Autodesk Inventor part; units mm, degrees
ref_plane "YZ Plane" through (0, 0, 0) normal (1, 0, 0) x (0, 1, 0)
ref_plane "XZ Plane" through (0, 0, 0) normal (0, 1, 0) x (-1, 0, 0)
ref_plane "XY Plane" through (0, 0, 0) normal (0, 0, 1) x (1, 0, 0)
sketch "Sketch1" plane through (0, 0, 0) normal (0, 1, 0) x (-1, 0, 0)
  circle A0 centre (0, 0) radius 7.25
  circle A1 centre (0, 0) radius 5.5
  dimension "d0" = 14.5
  dimension "d7" = 11
sketch "Sketch2" plane through (0, 0, 0) normal (0, 0, 1) x (1, 0, 0)
  line L0 (0, 0) -> (0, 23) construction
  line L1 (0, 23) -> (3, 23) construction
  line L2 (3, 23) -> (3, 46) construction
  spline S0 degree 3 poles (0, 0) (0, 23) (3, 23) (3, 46) knots 1 1 1 1 2 2 2 2
  line L3 (0, 46) -> (0, 0) construction
  line L4 (0, 46) -> (3, 46) construction
  dimension "d1" = 46
  dimension "d3" = 3
sweep "Sweep1" add profiles "Sketch1" path "Sketch2"
sketch "Sketch3" plane through (3, 46, 0) normal (0, 1, 0) x (1, 0, 0)
  circle A0 centre (-3, 0) radius 15
  circle A1 centre (-10.0711, 7.0711) radius 3.135
  circle A2 centre (-10.0711, -7.0711) radius 3.135
  circle A3 centre (-3, 0) radius 7.25 construction
  line L0 (-10.0711, 7.0711) -> (-3, 0) construction
  line L1 (-3, 0) -> (-18, 0) construction
  line L2 (-3, 0) -> (-10.0711, -7.0711) construction
  circle A4 centre (0, 0) radius 5.5
  point P0 (-10.25, 0)
  point P1 (-5.5, 0)
  dimension "d8" = 30
  dimension "d9" = 6.27
  dimension "d10" = 45
  dimension "d11" = 45
  dimension "d12" = 10
extrude "Extrusion1" add sketch "Sketch3" along normal blind 3
chamfer "Chamfer1" distance 1 angle 45 1 edges at (10.25, 46, 0)
chamfer "Chamfer2" distance 1 angle 45 1 edges at (-2.5, 49, 0)
properties part number "Nipple-3dprinted-metal" material "Stainless Steel"
Can you work these out from the model? Positions are in its coordinate system, mm. A direction names the side the tool comes from. Round coordinates to 2 decimals unless told otherwise and drop trailing zeros. Order: outer loops, then holes, each group sorted by start corner. A loop starts at its lowest first (then second) coordinate and runs counter-clockwise, first axis right, second up. Notation, with made-up numbers: (-40, 61) -> (-33, 61) arc R20 cw to (-33, 78) -> close; hole circle Ø8 at (20, 4). An arc over 180 degrees is marked (long way). Write each question's results on one line, items separated by ' | '. Start each with the question number.
Item 1: Which directions (+Z, -Z, +X, -X, +Y, -Y) give clear straight access to the entire face, cutting with the end or side of a thin tool? Please do faces 1 (the flat face through (-4, 49, 0)), 2 (the cylindrical face through (-4.08, 47.48, 8.01)).
Item 2: Please list where these lines run through material, in increasing order: L1, parallel to Y at x = 10.5, z = 6; L2, parallel to Z at x = 6.5, y = 30; L3, parallel to X at y = 19, z = -4.
Item 3: Thinking about a two-plate mould opening in X: for faces 3 (the flat face through (-7, 46, 0)), 4 (the cylindrical face through (-14.985, 47.479, 0.66)), 5 (the cylindrical face through (8.08, 46.99, -2.11)), which applies, +X half, -X half, draft (parallel to the pull), parting line (faces both ways), or undercut?
Item 4: Will these pins go through, and if not, where does the flat tip stop? pin 1 (10 mm diameter, centred on x = -7.07, z = -7.07, fed in from +Y); pin 2 (10 mm diameter, centred on y = 25.5, z = -2.5, fed in from +X); pin 3 (10 mm diameter, centred on x = 3, y = 26.5, fed in from +Z); pin 4 (1 mm diameter, centred on y = 34, z = 4, fed in from -X).
Item 5: If we section it at A-A, the plane z = 12: Write out the boundary of the cut face in (x, y).
Results:
1) face 1: +Z, -Z, +X, -X, +Y | face 2: +Y
2) L1: y = 46 to 49 | L2: z = -5.94 to -3.6, 3.6 to 5.94 | L3: x = -5.09 to -2.8, 4.8 to 7.09
3) face 3: draft | face 4: parting line | face 5: undercut
4) pin 1: stops at y = 49 | pin 2: stops at x = 9.6 | pin 3: stops at z = 7.25 | pin 4: stops at x = -3.72
5) outline: (-9, 46) -> (9, 46) -> (9, 49) -> (-9, 49) -> close
